Source: CAD feature listing. Evaluate the final solid. Frame: model axes, mm. A direction names the side the tool comes from. Round coordinates to 2 decimals unless told otherwise and drop trailing zeros. Loops run counter-clockwise (first coordinate to the right, second up) from the corner with the lowest first, then second, coordinate; pieces in that order, holes last. Notation, with made-up numbers: M 26,19 L 32,19 A26 ccw 32,52 Z; hole C 15,-32 d4. An arc over 180 degrees is marked long. One line per item, written item: value.
from build123d import *

# Parameters (mm, degrees)
SKETCH1_R           = 15
BOSS_EXTRUDE2_DEPTH = 100
SKETCH3_W           = 115
SKETCH3_H           = 30
BOSS_EXTRUDE3_DEPTH = 160
SKETCH4_W           = 5
SKETCH4_H           = 30
SKETCH4_W_2         = 105
CUT_EXTRUDE1_DEPTH  = 320
FILLET5_R           = 20
FILLET6_R           = 20
SKETCH6_W           = 8
SKETCH6_H           = 45
BOSS_EXTRUDE4_DEPTH = 80
CUT_EXTRUDE2_DEPTH  = 80


with BuildPart() as part:
    # Sketch1 → Boss-Extrude2 (new body)
    with BuildSketch(Plane.XY):
        with BuildLine():
            ThreePointArc((33.541666667, -109.999802714), (36.786992802, -108.957409847), (40, -107.819293264))
            Line((40, -107.819293264), (40, 107.819293264))
            ThreePointArc((40, 107.819293264), (0, 115), (-40, 107.819293264))
            Line((-40, 107.819293264), (-40, -107.819293264))
            ThreePointArc((-40, -107.819293264), (-36.786992802, -108.957409847), (-33.541666667, -109.999802714))
            ThreePointArc((-33.541666667, -109.999802714), (-30.981812183, -111.806807654), (-30, -114.782402832))
            Line((-30, -114.782402832), (-30, -145))
            ThreePointArc((-30, -145), (-35.857864376, -159.142135624), (-50, -165))
            Line((-50, -165), (-30, -165))
            Line((-30, -165), (30, -165))
            Line((30, -165), (50, -165))
            ThreePointArc((50, -165), (35.857864376, -159.142135624), (30, -145))
            Line((30, -145), (30, -114.782402832))
            ThreePointArc((30, -114.782402832), (30.981812183, -111.806807654), (33.541666667, -109.999802714))
        make_face()
        with Locations((0, -75)):
            Circle(SKETCH1_R, mode=Mode.SUBTRACT)
        with Locations((0, 75)):
            Circle(SKETCH1_R, mode=Mode.SUBTRACT)
    extrude(amount=BOSS_EXTRUDE2_DEPTH)

    # Sketch3 → Boss-Extrude3 (add, symmetric)
    with BuildSketch(Plane.XY):
        with Locations((0, -180)):
            Rectangle(SKETCH3_W, SKETCH3_H)
    extrude(amount=BOSS_EXTRUDE3_DEPTH, both=True)

    # Sketch4 → Cut-Extrude1 (cut)
    with BuildSketch(Plane(origin=(57.5, 0, 0), x_dir=(0, 0, -1), z_dir=(1, 0, 0))):
        with Locations((-157.5, -180)):
            Rectangle(SKETCH4_W, SKETCH4_H)
        with Locations((107.5, -180)):
            Rectangle(SKETCH4_W_2, SKETCH4_H)
    extrude(amount=-CUT_EXTRUDE1_DEPTH, mode=Mode.SUBTRACT)

    # Fillet5
    fillet5_edges = [part.edges().sort_by_distance(p)[0] for p in [
        (0, -165, 100),
    ]]
    fillet(fillet5_edges, radius=FILLET5_R)

    # Fillet6
    fillet6_edges = [part.edges().sort_by_distance(p)[0] for p in [
        (0, -165, 0),
    ]]
    fillet(fillet6_edges, radius=FILLET6_R)

    # Sketch6 → Boss-Extrude4 (add)
    with BuildSketch(Plane(origin=(40, 0, 0), x_dir=(0, 0, -1), z_dir=(1, 0, 0))):
        with Locations((4, 0)):
            Rectangle(SKETCH6_W, SKETCH6_H)
    extrude(amount=-BOSS_EXTRUDE4_DEPTH)

    # Sketch7 → Cut-Extrude2 (cut)
    with BuildSketch(Plane(origin=(40, 0, 0), x_dir=(0, 0, -1), z_dir=(1, 0, 0))):
        with BuildLine():
            Line((-40, 40), (-100, 40))
            Line((-100, 40), (-100, -40))
            Line((-100, -40), (-40, -40))
            ThreePointArc((-40, -40), (0, 0), (-40, 40))
        make_face()
    extrude(amount=-CUT_EXTRUDE2_DEPTH, mode=Mode.SUBTRACT)


solid = part.part
1. Section query D-D (y = 0). Return the cut outline in (x, z), and give its area (3 significant figures).
Report:
outline: M -40,-8 L 40,-8 L 40,0 L -40,0 Z
area: 640 mm2
2. Reachability of faces 1 (the face through (1, 22.5, -4)), 2 (the face through (-36.832, -108.942, 49.3)), 3 (the face through (1, -40, 70)), 4 (the face through (1, -22.5, -4)) from +Z, -Z, +X, -X, +Y, -Y: full face, straight path, thin tool, end or side. Return the list, or none.
Report:
face 1: -Z, +X, -X, +Y
face 2: +Z, -Z, -X
face 3: +Z, +X, -X
face 4: -Z, +X, -X
3. Section query A-A (y = 75). Return the cut outline in (x, z), and give its area (3 significant figures).
Report:
outline: M -40,0 L -15,0 L -15,100 L -40,100 Z; M 15,0 L 40,0 L 40,100 L 15,100 Z
area: 5,000 mm2
4. Pin query (flat end, axial travel): pin 1 (24 mm diameter, centred on y = -127.5, z = 74.5, fed in from +X); pin 2 (8 mm diameter, centred on x = 14.5, y = 62, fed in from -Z); pin 3 (18 mm diameter, centred on x = 0, y = -75, fed in from -Z); pin 4 (8 mm diameter, centred on x = -12, z = 18, fed in from +Y). Return the tip coordinate at first contact, or that it passes through.
Report:
pin 1: stops at x = 30
pin 2: stops at z = 0
pin 3: passes through
pin 4: stops at y = 114.72
5. Pull-direction query (Y, two-part tool) for faces 5 (the face through (-35.703, -158.986, 49.02)), 6 (the face through (-1, -195, 51)), 7 (the face through (-1, 95, 100)); classes: released by +Y, released by -Y, zero draft, split by the parting line, or undercut.
Report:
face 5: undercut
face 6: released by -Y
face 7: zero draft
6. Section query C-C (x = 0). Return the cut outline in (y, z), and give its area (3 significant figures).
Report:
outline: M -195,-55 L -165,-55 L -165,-20 A20 cw -145,0 L -90,0 L -90,100 L -145,100 A20 cw -165,120 L -165,155 L -195,155 Z; M -60,0 L -22.5,0 L -22.5,-8 L 22.5,-8 L 22.5,0 L 60,0 L 60,100 L 40,100 L 40,40 A40 cw -40,40 L -40,100 L -60,100 Z; M 90,0 L 115,0 L 115,100 L 90,100 Z
area: 21,500 mm2
7. Section query B-B (z = 14). Return the cut outline in (x, y).
Report:
outline: M -57.5,-195 L 57.5,-195 L 57.5,-165 L 50,-165 A20 cw 30,-145 L 30,-114.78 A5 cw 33.54,-110 A115 ccw 40,-107.82 L 40,-30.4 L -40,-30.4 L -40,-107.82 A115 ccw -33.54,-110 A5 cw -30,-114.78 L -30,-145 A20 cw -50,-165 L -57.5,-165 Z; M -40,30.4 L 40,30.4 L 40,107.82 A115 ccw -40,107.82 Z; hole C 0,-75 d30; hole C 0,75 d30
8. Ray query, line 1 (Y direction, x = 0, z = 38); line 2 (Y direction, x = 0, z = 70); line 3 (Y direction, x = -52, z = -34.5). Return the intervals inside material, ascending. Write a range as [from, to].
Report:
line 1: y = [-195, -90], [-60, -39.95], [39.95, 60], [90, 115]
line 2: y = [-195, -90], [-60, -40], [40, 60], [90, 115]
line 3: y = [-195, -165]
